Autodesk Fusion 360 part; units mm, degrees
sketch "草图1" plane through (0, 0, 0) normal (0, 0, 1) x (1, 0, 0)
  line L0 (0, 0) -> (14.8, 0)
  line L1 (14.8, 0) -> (14.8, 7.8)
  line L2 (14.8, 7.8) -> (0, 7.8)
  line L3 (0, 7.8) -> (0, 0)
  arc A0 (0, 2.7439) -> (0, 5.026) centre (1.1216, 3.885) ccw
  dimension "d1" = 14.8
  dimension "d2" = 7.8
  dimension "d3" = 3.2
extrude "拉伸1" add sketch "草图1" along normal blind 5 contours L0 L1 L2 L3 A0
sketch "草图2" plane through (0, 0, 5) normal (0, 0, 1) x (-1, 0, 0)
  line L0 (0, 0) -> (-14.8, 0)
  line L1 (-14.8, 0) -> (-14.8, -7.8)
  line L2 (-14.8, -7.8) -> (0, -7.8)
  line L3 (0, -7.8) -> (0, -5.026)
  arc A0 (0, -2.7439) -> (0, -5.026) centre (-1.1216, -3.885) ccw
  line L4 (0, -2.7439) -> (0, 0)
  line L5 (3, -10.0312) -> (-17.9802, -10.0312)
  line L6 (-17.9802, -10.0312) -> (-17.9802, 1.9802)
  line L7 (-17.9802, 1.9802) -> (3, 1.9802)
  line L8 (3, 1.9802) -> (3, -10.0312)
extrude "拉伸2" add sketch "草图2" along normal blind 2 contours L0 L1 L2 L3 A0 L4 | L5 L6 L7 L8
extrude "拉伸3" cut sketch "草图1" along normal blind 13 contours L3 A0
sketch "草图3" plane through (0, 0, 5) normal (0, 0, -1) x (1, 0, 0)
  line L0 (0, -5.026) -> (0, -2.7439)
  line L1 (0, -2.7439) -> (0, 0)
  line L2 (0, 0) -> (14.8, 0)
  line L3 (14.8, 0) -> (14.8, -7.8)
  line L4 (14.8, -7.8) -> (0, -7.8)
  line L5 (0, -7.8) -> (0, -5.026)
  line L6 (17.9802, 1.9802) -> (-3, 1.9802)
  line L7 (-3, 1.9802) -> (-3, -10.0312)
  line L8 (-3, -10.0312) -> (17.9802, -10.0312)
  line L9 (17.9802, -10.0312) -> (17.9802, 1.9802)
  line L10 (0, -2.7439) -> (-3, -2.7439)
  line L11 (0, -5.026) -> (-3, -5.026)
extrude "拉伸4" cut sketch "草图3" against normal blind 2 contours L0 L7 L10 L11
Read the model definition and answer for the solid it produces. Units are mm, in the model's axes. A direction names the side the tool comes from. Give positions to 0.01 mm unless a question says otherwise; leave off trailing zeros. Order: outer loops, then holes, each group sorted by start corner. A loop starts at its lowest first (then second) coordinate and runs counter-clockwise, first axis right, second up. Notation, with made-up numbers: (28, 22) -> (39, 22) arc R15 ccw to (39, 27) -> close; hole circle Ø5 at (-6.5, 36.5). An arc over 180 degrees is marked (long way). Write item = value, one per line.
1. The mould has two halves that part along Y. Classify faces 5 (the face through (0, 1, 2)), 6 (the face through (2.72, 3.94, 3.45)), 7 (the face through (8, 7.8, 2)): +Y half, -Y half, draft (parallel to the pull), parting line (faces both ways), or undercut.
Numbers:
face_5 = draft
face_6 = undercut
face_7 = +Y half
2. A cutting plane is placed at D-D, the plane z = 1.75. Write down the section's boundary in (x, y), and give its area (3 significant figures).
Numbers:
outline = (0, 0) -> (14.8, 0) -> (14.8, 7.8) -> (0, 7.8) -> (0, 5.03) arc R1.6 cw (long way) to (0, 2.74) -> close
area = 108 mm²
3. A cutting plane is placed at A-A, the plane x = 9.25. Write down the section's boundary in (y, z).
Numbers:
outline = (-1.98, 5) -> (0, 5) -> (0, 0) -> (7.8, 0) -> (7.8, 5) -> (10.03, 5) -> (10.03, 7) -> (-1.98, 7) -> close
4. Straight lines are drawn through the part: line 1 along Z through (x, y) = (1.5, -0.25); line 2 along X through (y, z) = (6.75, 1.75); line 3 along Y through (x, z) = (1.5, 3). For each, find the intervals that lie inside material, in ascending order.
Numbers:
line_1 = 5 to 7
line_2 = 0 to 14.8
line_3 = 0 to 2.33, 5.44 to 7.8
5. For faces 1 (the face through (0, 6, 2)), 2 (the face through (14.8, 4, 2)), 3 (the face through (-1, 5.026, 6)), 4 (the face through (7, 0, 2)), determine the directions among +Z, -Z, +X, -X, +Y, -Y from which every point of the face is accessible in a straight line to the end or side of a thin tool.
Numbers:
face_1 = -Z, -X, +Y, -Y
face_2 = -Z, +X, +Y, -Y
face_3 = +Z, -Z, -X
face_4 = -Z, +X, -X, -Y
6. Given pin 1 (1.4 mm diameter, centred on y = 6.5, z = 1.5, fed in from -X); pin 2 (2.5 mm diameter, centred on x = 10, z = 3.5, fed in from +Y); pin 3 (4 mm diameter, centred on y = 4.5, z = 2, fed in from +X), each flat-ended and moving along its own axis, determine where each tip first touches the part or whether it passes through.
Numbers:
pin_1 = 0
pin_2 = 7.8
pin_3 = 14.8
7. A cutting plane is placed at C-C, the plane x = 2.5. Write down the section's boundary in (y, z), and give its area (3 significant figures).
Numbers:
outline = (-1.98, 5) -> (0, 5) -> (0, 0) -> (3.07, 0) -> (3.07, 7) -> (-1.98, 7) -> close; (4.7, 0) -> (7.8, 0) -> (7.8, 5) -> (10.03, 5) -> (10.03, 7) -> (4.7, 7) -> close
area = 51.6 mm²
8. A cutting plane is placed at B-B, the plane y = 7.5. Write down the section's boundary in (x, z), and give its area (3 significant figures).
Numbers:
outline = (-3, 5) -> (0, 5) -> (0, 0) -> (14.8, 0) -> (14.8, 5) -> (17.98, 5) -> (17.98, 7) -> (-3, 7) -> close
area = 116 mm²
